For this review, take the finished solid that the model builds, in its own axes (mm). A direction names the side the tool comes from. Coordinates: 2 decimals unless noted, no trailing zeros. Loops run counter-clockwise (first coordinate to the right, second up) from the corner with the lowest first, then second, coordinate; pieces in that order, holes last. Notation, with made-up numbers: (46.25, 12.25) -> (102.25, 12.25) arc R15 cw to (102.25, 23.25) -> close; hole circle Ø11 at (-31, 34). An arc over 180 degrees is marked (long way). Use a Markdown table: item, result.
from build123d import *

# Parameters (mm, degrees)
F_3DSKETCH1_R       = 6
BOSS_EXTRUDE3_DEPTH = 3
SKETCH3_R           = 7.5
SKETCH3_R_2         = 5
BOSS_EXTRUDE5_DEPTH = 19


with BuildPart() as part:
    # 3DSketch1 → Boss-Extrude3 (new body)
    with BuildSketch(Plane(origin=(-1.906972696, 0, 4.753867784), x_dir=(0.8585635359116023, 0, 0.5127071823204421), z_dir=(0, -1, 0))):
        Polygon((0, 0), (9.634447543, 16.133546855), (36.65118441, 0), (27.016736867, -16.133546855), align=None)
        with Locations(Location((23.762707279, -3.079667236, 0), (0, 0, 59.155677363))):
            Circle(F_3DSKETCH1_R, mode=Mode.SUBTRACT)
    extrude(amount=-BOSS_EXTRUDE3_DEPTH)

    # Sketch3 → Boss-Extrude5 (add)
    with BuildSketch(Plane(origin=(-8.525652269, 0, 23.545193271), x_dir=(1, 0, 0), z_dir=(0, 0, 1))):
        with Locations((-0.242866193, 0)):
            Circle(SKETCH3_R)
        Circle(SKETCH3_R_2, mode=Mode.SUBTRACT)
    extrude(amount=-BOSS_EXTRUDE5_DEPTH)


solid = part.part
(1) Take a section at B-B on x = -11.5. Write out the cut boundary in (y, z).
Found:
| item | result |
|---|---|
| outline | (-6.98, 4.55) -> (-4.02, 4.55) -> (-4.02, 23.55) -> (-6.98, 23.55) -> close; (4.02, 4.55) -> (6.98, 4.55) -> (6.98, 23.55) -> (4.02, 23.55) -> close |
(2) For line 1 along X through (y, z) = (1.25, 14); line 2 along Y through (x, z) = (9.5, 18); line 3 along Z through (x, y) = (26.5, 0.25), list the stretches that pass through material, from the lowest coordinate up.
Found:
| item | result |
|---|---|
| line 1 | x = -16.16 to -13.37, -3.68 to 14.08, 26.07 to 29.56 |
| line 2 | y = 0 to 3 |
| line 3 | z = 4.75 to 23.55 |
(3) Take a section at D-D on z = 6. Write out the cut boundary in (x, y).
Found:
| item | result |
|---|---|
| outline | (-1.89, 3) arc R7.5 ccw (long way) to (-1.27, 0) -> (29.56, 0) -> (29.56, 3) -> close; hole circle Ø10 at (-8.53, 0) |
(4) For faces 5 (the face through (13.9, 3, 14.5)), 6 (the face through (-14, 0, 4.545)), 7 (the face through (11, 0, 12)), list the 3-axis set-ups (+Z, -Z, +X, -X, +Y, -Y) from which the entire face can be reached by the end or side of a thin tool; tool diameter is ignored.
Found:
| item | result |
|---|---|
| face 5 | +Z, -Z, +X, +Y |
| face 6 | -Z, +X, -X, +Y, -Y |
| face 7 | +Z, -Z, +X, -Y |
(5) Mouldability with a two-part tool opening along X and no side actions: class faces 1 (the face through (-13.52, 0.22, 14.18)), 2 (the face through (29.56, 1, 14)), 3 (the face through (-16.26, 0.33, 14.18)), 4 (the face through (14, 1, 4.754)) as pulls with the +X half, pulls with the -X half, needs draft (parallel to the pull), parting line crosses it, or undercut.
Found:
| item | result |
|---|---|
| face 1 | undercut |
| face 2 | pulls with the +X half |
| face 3 | parting line crosses it |
| face 4 | needs draft |
(6) Take a section at C-C on y = 3.75. Write out the cut boundary in (x, z), plus the area to 3 significant figures.
Found:
| item | result |
|---|---|
| outline | (-15.26, 4.55) -> (-11.83, 4.55) -> (-11.83, 23.55) -> (-15.26, 23.55) -> close; (-5.22, 4.55) -> (-2.27, 4.55) -> (-2.27, 23.55) -> (-5.22, 23.55) -> close |
| area | 121 mm^2 |
(7) Take a section at A-A on z = 11.5. Write out the cut boundary in (x, y), plus the area to 3 significant figures.
Found:
| item | result |
|---|---|
| outline | (-1.89, 3) arc R7.5 ccw (long way) to (-1.27, 0) -> (14.76, 0) -> (14.76, 3) -> close; (25.38, 0) -> (29.56, 0) -> (29.56, 3) -> (25.38, 3) -> close; hole circle Ø10 at (-8.53, 0) |
| area | 159 mm^2 |
(8) For pin 1 Ø3.5 at (x, y) = (7.5, 1) entering from -Z; pin 2 Ø6 at (x, z) = (7, 19) entering from -Y; pin 3 Ø2 at (y, z) = (-4.5, 20) entering from -X; pin 4 Ø9 at (x, y) = (-8.53, 0) entering from +Z, all flat-tipped, find the tip position at first contact; note any pin that passes through.
Found:
| item | result |
|---|---|
| pin 1 | stops at z = 4.75 |
| pin 2 | stops at y = 0 |
| pin 3 | stops at x = -15.4 |
| pin 4 | passes through |
